Input: part model. Units: mm. Frame: model coordinates. A direction names the side the tool comes from. Round coordinates to 2 decimals unless told otherwise and drop trailing zeros. Loops run counter-clockwise (first coordinate to the right, second up) from the corner with the lowest first, then second, coordinate; pieces in that order, holes last. Notation, with made-up numbers: (29, 22) -> (70, 22) arc R8 ccw to (70, 26) -> close; hole circle Ø3 at (80, 12.5). An arc over 180 degrees is marked (long way). Answer in a Markdown table with one row per item. Add a question column.
Q1. Section D-D, the plane x = 76.65. Output: boundary loops of the cut face in (y, z).
Q2. Reachability of faces 1 (the face through (130, 62, 2.5)), 2 (the face through (114, 56, 5)), 3 (the face through (26.15, 45, 2)), 4 (the face through (154, 54.7, -3.8)) from +Z, -Z, +X, -X, +Y, -Y: full face, straight path, thin tool, end or side. Return the list, or none.
Q3. Section B-B, the plane y = 43. Output: boundary loops of the cut face in (x, z).
Q4. Pin query (flat end, axial travel): pin 1 (8 mm diameter, centred on x = 11.75, y = 48.57, fed in from -Z); pin 2 (6 mm diameter, centred on x = 120.12, y = 22.1, fed in from +Z); pin 3 (7 mm diameter, centred on y = 40.5, z = -10, fed in from -X); pin 4 (7 mm diameter, centred on x = 76.65, y = 13.63, fed in from -Z). Return the tip coordinate at first contact, or that it passes through.
Q5. Ray query, L1, parallel to X at y = 13.63, z = 1.4; L2, parallel to Y at x = 86.95, z = 2.4; L3, parallel to Y at x = 130.08, z = 1.55. Return the intervals inside material, ascending. Write a range as from..to.
Q6. Section C-C, the plane z = -7. Output: boundary loops of the cut face in (x, y).
Q7. Section A-A, the plane x = 19. Output: boundary loops of the cut face in (y, z).
Q8. Mould query, pull axis Y, two halves, no side actions, for faces 5 (the face through (156.5, 52.5, -6.9)), 6 (the face through (110, 56, 0)). Classes: pulls with the +Y half, pulls with the -Y half, needs draft (parallel to the pull), parting line crosses it, or undercut.
```python
from build123d import *

# Parameters (mm, degrees)
F0_W     = 159
F0_H     = 111
F0_R     = 2.5
F0_R_2   = 2
F1_DEPTH = 5
F2_W     = 5
F2_H     = 111
F3_DEPTH = 19
F4_R     = 3
F5_DEPTH = 5
F6_R     = 6
F7_DEPTH = 2.5


with BuildPart() as f1:
    # F0 (on Top) → F1 (new body)
    with BuildSketch(Plane.XY):
        with Locations((79.5, 55.5)):
            Rectangle(F0_W, F0_H)
        with Locations((11.75, 48.57)):
            Circle(F0_R, mode=Mode.SUBTRACT)
        with Locations((120.12, 22.1)):
            Circle(F0_R, mode=Mode.SUBTRACT)
        with Locations((6, 76)):
            Circle(F0_R_2, mode=Mode.SUBTRACT)
        Polygon((16.15, 62.95), (16.15, 89.95), (102.15, 89.95), (102.15, 26.95), (26.15, 26.95), (26.15, 62.95), align=None, mode=Mode.SUBTRACT)
        with Locations((86.95, 93.97)):
            Circle(F0_R, mode=Mode.SUBTRACT)
    extrude(amount=F1_DEPTH)

    # F2 (on face) → F3 (join)
    with BuildSketch(Plane.XY.offset(5)):
        with Locations((156.5, 55.5)):
            Rectangle(F2_W, F2_H)
    extrude(amount=-F3_DEPTH)

    # F4 (on face) → F5 (cut)
    with BuildSketch(Plane.YZ.offset(159)):
        with Locations((55.5, -7)):
            Circle(F4_R)
    extrude(amount=-F5_DEPTH, mode=Mode.SUBTRACT)

    # F6 (on face) → F7 (cut)
    with BuildSketch(Plane(origin=(0, 0, 0), x_dir=(1, 0, 0), z_dir=(0, 0, -1))):
        with Locations((76.65, -13.63)):
            Circle(F6_R)
        with Locations((130.08, -62.15)):
            Circle(F6_R)
        with Locations((40.11, -99.03)):
            Circle(F6_R)
    extrude(amount=-F7_DEPTH, mode=Mode.SUBTRACT)


solid = f1.part
```
Answer block:
| question | item | result |
|---|---|---|
| 1 | outline | (0, 0) -> (7.63, 0) -> (7.63, 2.5) -> (19.63, 2.5) -> (19.63, 0) -> (26.95, 0) -> (26.95, 5) -> (0, 5) -> close; (89.95, 0) -> (111, 0) -> (111, 5) -> (89.95, 5) -> close |
| 2 | face 1 | -Z |
| 2 | face 2 | +Z, +X, -X, +Y, -Y |
| 2 | face 3 | +Z, -Z |
| 2 | face 4 | -Z, -X, +Y, -Y |
| 3 | outline | (0, 0) -> (26.15, 0) -> (26.15, 5) -> (0, 5) -> close; (102.15, 0) -> (154, 0) -> (154, -14) -> (159, -14) -> (159, 5) -> (102.15, 5) -> close |
| 4 | pin 1 | z = 0 |
| 4 | pin 2 | z = 5 |
| 4 | pin 3 | x = 154 |
| 4 | pin 4 | z = 2.5 |
| 5 | L1 | 0..70.65, 82.65..159 |
| 5 | L2 | 0..26.95, 89.95..91.47, 96.47..111 |
| 5 | L3 | 0..56.15, 68.15..111 |
| 6 | outline | (154, 0) -> (159, 0) -> (159, 52.5) -> (154, 52.5) -> close; (154, 58.5) -> (159, 58.5) -> (159, 111) -> (154, 111) -> close |
| 7 | outline | (0, 0) -> (62.95, 0) -> (62.95, 5) -> (0, 5) -> close; (89.95, 0) -> (111, 0) -> (111, 5) -> (89.95, 5) -> close |
| 8 | face 5 | undercut |
| 8 | face 6 | needs draft |
